Source: CAD feature listing. Evaluate the final solid. Frame: model axes, mm. Face numbers are marked on the shaded views. A direction names the side the tool comes from. Give positions to 0.01 mm unless a question says otherwise; leave off trailing zeros. Order: outer loops, then holes, each group sorted by start corner. A loop starts at its lowest first (then second) coordinate and runs counter-clockwise, first axis right, second up. Notation, with made-up numbers: M 58.5,49.25 L 76.5,49.25 A19 ccw 76.5,67.25 Z; hole C 68.25,29.25 d6. An arc over 180 degrees is marked long. Use CSV: the item, a comma, the result in double quotes. Start each with the question number.
Item 1: Section query C-C on z = 3.5. Return loops of the section in (x, y), and give its area (3 significant figures).
Item 2: Access query for the marked faces 1 and 2. Directions: +Z, -Z, +X, -X, +Y, -Y. A direction counts if a zero-diameter tool reaches every point of the face in a straight line with its end or side. Return the directions, or none.
Item 3: Ray query, probe 1 along Y at (x, z) = (0, -1.25); probe 2 along X at (y, z) = (-28, 1.75); probe 3 along Y at (x, z) = (8, -2). Return the intervals inside material, ascending. Write a range as from..to.
Item 4: Section query B-B on x = 0. Return loops of the section in (y, z), and give its area (3 significant figures).
Item 5: Section query D-D on x = -12. Return loops of the section in (y, z).
Item 6: Pull-direction query (Y, two-part tool) for the marked faces 3, 4 and 5; classes: +Y half, -Y half, draft (parallel to the pull), parting line (faces both ways), or undercut.
Item 7: First-contact query: pin 1 (5 mm diameter, centred on y = -26.5, z = -0.5, fed in from -X); pin 2 (1.5 mm diameter, centred on x = 24, z = 1.5, fed in from +Y); pin 3 (3 mm diameter, centred on y = 2, z = 0.5, fed in from +X). Flat tips, straight axial feed; report the tip coordinate or a pass-through.
Item 8: Section query A-A on y = 0. Return loops of the section in (x, z), and give its area (3 significant figures).
from build123d import *

# Parameters (mm, degrees)
SKETCH1_R           = 15
BOSS_EXTRUDE1_DEPTH = 5
SKETCH2_R           = 4
CUT_EXTRUDE1_DEPTH  = 62.23724357


with BuildPart() as part:
    # Sketch1 → Boss-Extrude1 (new, symmetric)
    with BuildSketch(Plane.XY):
        with BuildLine():
            Line((-40.311288741, 20), (-17.91612833, 8.888888889))
            ThreePointArc((-17.91612833, 8.888888889), (-18.699713239, -7.093710227), (-7.512794536, -18.535315435))
            Line((-7.512794536, -18.535315435), (-7.512794536, -44.368433804))
            ThreePointArc((-7.512794536, -44.368433804), (0, -45), (7.512794536, -44.368433804))
            Line((7.512794536, -44.368433804), (7.512794536, -18.535315435))
            ThreePointArc((7.512794536, -18.535315435), (18.699713239, -7.093710227), (17.91612833, 8.888888889))
            Line((17.91612833, 8.888888889), (40.311288741, 20))
            ThreePointArc((40.311288741, 20), (0, 45), (-40.311288741, 20))
        make_face()
        Circle(SKETCH1_R, mode=Mode.SUBTRACT)
    extrude(amount=BOSS_EXTRUDE1_DEPTH, both=True)

    # Sketch2 → Cut-Extrude1 (cut, through all)
    with BuildSketch(Plane.XY.offset(5)):
        with Locations((0, -40)):
            Circle(SKETCH2_R)
    extrude(amount=-CUT_EXTRUDE1_DEPTH, mode=Mode.SUBTRACT)


solid = part.part
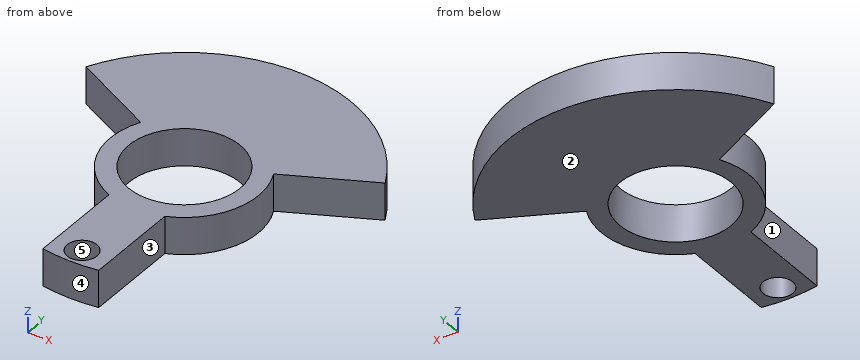
Verdict:
1,outline,"M -40.31,20 L -17.92,8.89 A20 ccw -7.51,-18.54 L -7.51,-44.37 A45 ccw 7.51,-44.37 L 7.51,-18.54 A20 ccw 17.92,8.89 L 40.31,20 A45 ccw Z; hole C 0,0 d30; hole C 0,-40 d8"
1,area,"2,680 mm2"
2,face 1,"+Z, -Z, -X, -Y"
2,face 2,"-Z, +X, -X, +Y, -Y"
3,probe 1,"-45..-44, -36..-15, 15..45"
3,probe 2,"-7.51..7.51"
3,probe 3,"-18.33..-12.69, 12.69..44.28"
4,outline,"M -45,-5 L -44,-5 L -44,5 L -45,5 Z; M -36,-5 L -15,-5 L -15,5 L -36,5 Z; M 15,-5 L 45,-5 L 45,5 L 15,5 Z"
4,area,"520 mm2"
5,outline,"M -16,-5 L -9,-5 L -9,5 L -16,5 Z; M 9,-5 L 43.37,-5 L 43.37,5 L 9,5 Z"
6,face 3,"draft"
6,face 4,"-Y half"
6,face 5,"undercut"
7,pin 1,"x = -7.51"
7,pin 2,"y = 38.53"
7,pin 3,"x = 19.99"
8,outline,"M -20,-5 L -15,-5 L -15,5 L -20,5 Z; M 15,-5 L 20,-5 L 20,5 L 15,5 Z"
8,area,"100 mm2"
